Study the drawing (mm; zero at the part's minimum x, y, z) and answer. A direction names the side the tool comes from. Coordinates: 2 decimals unless noted, no trailing zeros. Loops run counter-clockwise (first coordinate to the right, second up) from the corner with the lowest first, then second, coordinate; pieces in that order, holes last. Notation, with made-up numbers: (-25.75, -24) -> (-19.75, -24) arc R16 cw to (-19.75, -6) -> close; hole circle Ø5 at (10.5, 29.5). An arc over 180 degrees is marked (long way). Answer as a JSON object with one key per item and string values. Group by question number.
Q1. Straight lines are drawn through the part: line 1 along Z through (x, y) = (35, 9.75); line 2 along X through (y, z) = (8.75, 16.5); line 3 along Z through (x, y) = (108, 2.5). For each, find the intervals that lie inside material, in ascending order. Write a range as [from, to].
Q2. The part is cut by section B-B on y = 13.75. Write down the section's boundary in (x, z).
Q3. The part is cut by section A-A on x = 104. Write down the section's boundary in (y, z).
Q4. For the marked faces 1 and 2, determine the directions among +Z, -Z, +X, -X, +Y, -Y from which every point of the face is accessible in a straight line to the end or side of a thin tool.
Q5. The part is cut by section C-C on z = 29.95. Write down the section's boundary in (x, y).
Q6. Each of these flat-tipped pins is pushed along its axis until it touches: P1, Ø7.5, axis at y = 4, z = 32.5, coming from the +X side; P2, Ø17.5, axis at x = 35, z = 29.95, coming from the +Y side. Where does it stop, or does it pass through?
Q7. The part is cut by section D-D on z = 16. Write down the section's boundary in (x, y), and give its area (4 significant figures).
Q8. Determine the mould class of the marked faces 3, 4 and 5 for opening direction X: released by +X, released by -X, zero draft, split by the parting line, or undercut.
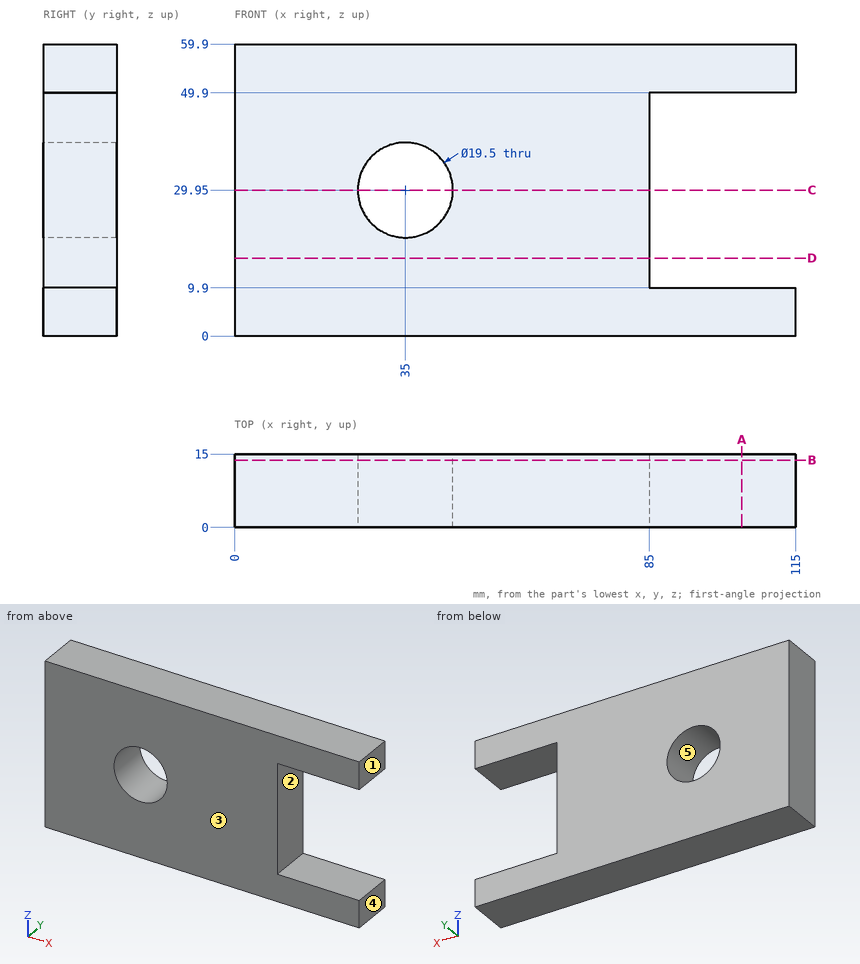
Final values:
{
 "1": {"line 1": "z = [0, 20.2], [39.7, 59.9]", "line 2": "x = [0, 85]", "line 3": "z = [0, 9.9], [49.9, 59.9]"},
 "2": {"outline": "(0, 0) -> (115, 0) -> (115, 9.9) -> (85, 9.9) -> (85, 49.9) -> (115, 49.9) -> (115, 59.9) -> (0, 59.9) -> close; hole circle Ø19.5 at (35, 29.95)"},
 "3": {"outline": "(0, 0) -> (15, 0) -> (15, 9.9) -> (0, 9.9) -> close; (0, 49.9) -> (15, 49.9) -> (15, 59.9) -> (0, 59.9) -> close"},
 "4": {"face 1": "+Z, -Z, +X, +Y, -Y", "face 2": "+X, +Y, -Y"},
 "5": {"outline": "(0, 0) -> (25.25, 0) -> (25.25, 15) -> (0, 15) -> close; (44.75, 0) -> (85, 0) -> (85, 15) -> (44.75, 15) -> close"},
 "6": {"P1": "stops at x = 85", "P2": "passes through"},
 "7": {"outline": "(0, 0) -> (85, 0) -> (85, 15) -> (0, 15) -> close", "area": "1,275 mm2"},
 "8": {"face 3": "zero draft", "face 4": "released by +X", "face 5": "undercut"}
}
